from build123d import *

# Parameters (mm, degrees)
ESQUISSE3_R                  = 50
ESQUISSE3_R_2                = 42.5
BOSS_EXTRU_2_DEPTH           = 18
BOSS_EXTRU_3_START           = 3
ESQUISSE4_R                  = 50
BOSS_EXTRU_3_DEPTH           = 3
ESQUISSE5_R                  = 14
BOSS_EXTRU_4_DEPTH           = 7.5
BOSS_EXTRU_5_DEPTH           = 45
BOSS_EXTRU_5_DEPTH_BACK      = 45
CONG_1_R                     = 2
ESQUISSE6_R                  = 3.5
ENL_V_MAT_EXTRU_1_DEPTH      = 85.356386836
ESQUISSE7_R                  = 2
ENL_V_MAT_EXTRU_2_DEPTH      = 89.669329534
ENL_V_MAT_EXTRU_3_DEPTH      = 83.758685345
ENL_V_MAT_EXTRU_3_DEPTH_BACK = 4
ESQUISSE8_R                  = 3.5
ESQUISSE11_W                 = 24.696960071
ESQUISSE11_H                 = 3
BOSS_EXTRU_6_DEPTH           = 43
ENL_V_MAT_EXTRU_4_DEPTH      = 43
ESQUISSE13_R                 = 1.5
ENL_V_MAT_EXTRU_5_DEPTH      = 100.724620832
CHANFREIN1_SIZE              = 2
CHANFREIN2_SIZE              = 1.5


with BuildPart() as part:
    # Esquisse3 → Boss.-Extru.2 (new body)
    with BuildSketch(Plane(origin=(0, 0, 0), x_dir=(0, 0, -1), z_dir=(1, 0, 0))):
        Circle(ESQUISSE3_R)
        Circle(ESQUISSE3_R_2, mode=Mode.SUBTRACT)
    extrude(amount=BOSS_EXTRU_2_DEPTH)

    # Esquisse4 → Boss.-Extru.3 (add)
    with BuildSketch(Plane.ZY.offset(BOSS_EXTRU_3_START)):
        Circle(ESQUISSE4_R)
    extrude(amount=-BOSS_EXTRU_3_DEPTH)

    # Esquisse5 → Boss.-Extru.4 (add)
    with BuildSketch(Plane(origin=(0, 0, 0), x_dir=(0, 0, -1), z_dir=(1, 0, 0))):
        with Locations(Location((0, 0, 0), (0, 0, 180))):
            Circle(ESQUISSE5_R)
    extrude(amount=BOSS_EXTRU_4_DEPTH)

    # Esquisse10 → Boss.-Extru.5 (add, two sides: drawn at the far end of the back side and taken through both)
    with BuildSketch(Plane(origin=(0, 0, 0), x_dir=(1, 0, 0), z_dir=(0, 1, 0)).offset(-BOSS_EXTRU_5_DEPTH_BACK)):
        Polygon((-46, 23), (-3, 23), (-3, 20), (-43, 20), (-43, -20), (-3, -20), (-3, -23), (-46, -23), align=None)
    extrude(amount=BOSS_EXTRU_5_DEPTH + BOSS_EXTRU_5_DEPTH_BACK)

    # Congé1
    # the kernel refuses this fillet: 2 mm, written as the material it takes off along each edge
    with BuildSketch(Plane(origin=(-51, -45, -23), x_dir=(0, 0, 1), z_dir=(1, 0, 0)), Plane(origin=(-3, 45, 23), x_dir=(0, -1, 0), z_dir=(-1, 0, 0))) as cong_1_piece_1:
        with BuildLine():
            CenterArc((CONG_1_R, -CONG_1_R), CONG_1_R, 90, 90)
            Line((0, -CONG_1_R), (0, 0))
            Line((0, 0), (CONG_1_R, 0))
        make_face()
    extrude(amount=48, mode=Mode.SUBTRACT)
    with BuildSketch(Plane(origin=(-3, -45, 23), x_dir=(0, 1, 0), z_dir=(-1, 0, 0)), Plane(origin=(-51, 45, -23), x_dir=(0, 0, 1), z_dir=(1, 0, 0))) as cong_1_piece_2:
        with BuildLine():
            CenterArc((CONG_1_R, CONG_1_R), CONG_1_R, 180, 90)
            Line((0, CONG_1_R), (0, 0))
            Line((0, 0), (CONG_1_R, 0))
        make_face()
    extrude(amount=48, mode=Mode.SUBTRACT)

    # Esquisse6 → Enlèv. mat.-Extru.1 (cut, through all)
    with BuildSketch(Plane(origin=(0, 0, 0), x_dir=(0, 0, -1), z_dir=(1, 0, 0))):
        with Locations((-12.374368671, 12.374368671)):
            Circle(ESQUISSE6_R)
        with Locations((12.374368671, 12.374368671)):
            Circle(ESQUISSE6_R)
        with Locations((12.374368671, -12.374368671)):
            Circle(ESQUISSE6_R)
        with Locations((-12.374368671, -12.374368671)):
            Circle(ESQUISSE6_R)
    extrude(amount=-ENL_V_MAT_EXTRU_1_DEPTH, mode=Mode.SUBTRACT)

    # Esquisse7 → Enlèv. mat.-Extru.2 (cut, through all)
    with BuildSketch(Plane(origin=(7.5, 0, 0), x_dir=(0, 0, -1), z_dir=(1, 0, 0))):
        with Locations((0, 8.5)):
            Circle(ESQUISSE7_R)
        with Locations((7.361215932, 4.25)):
            Circle(ESQUISSE7_R)
        with Locations((7.361215932, -4.25)):
            Circle(ESQUISSE7_R)
        with Locations((0, -8.5)):
            Circle(ESQUISSE7_R)
        with Locations((-7.361215932, -4.25)):
            Circle(ESQUISSE7_R)
        with Locations((-7.361215932, 4.25)):
            Circle(ESQUISSE7_R)
    extrude(amount=-ENL_V_MAT_EXTRU_2_DEPTH, mode=Mode.SUBTRACT)

    # Esquisse8 → Enlèv. mat.-Extru.3 (cut, two sides: drawn at the far end of the back side and taken through both)
    with BuildSketch(Plane.ZY.offset(3).offset(-ENL_V_MAT_EXTRU_3_DEPTH_BACK)):
        with Locations((0, -8.5)):
            Circle(ESQUISSE8_R)
        with Locations((7.361215932, -4.25)):
            Circle(ESQUISSE8_R)
        with Locations((0, 8.5)):
            Circle(ESQUISSE8_R)
        with Locations((7.361215932, 4.25)):
            Circle(ESQUISSE8_R)
        with Locations((-7.361215932, -4.25)):
            Circle(ESQUISSE8_R)
        with Locations((-7.361215932, 4.25)):
            Circle(ESQUISSE8_R)
    extrude(amount=ENL_V_MAT_EXTRU_3_DEPTH + ENL_V_MAT_EXTRU_3_DEPTH_BACK, mode=Mode.SUBTRACT)

    # Esquisse11 → Boss.-Extru.6 (add)
    with BuildSketch(Plane.ZY.offset(3)):
        with Locations((35.348480036, 13.5)):
            Rectangle(ESQUISSE11_W, ESQUISSE11_H)
        with Locations((35.348480036, -13.5)):
            Rectangle(ESQUISSE11_W, ESQUISSE11_H)
        with Locations((-35.348480036, -13.5)):
            Rectangle(ESQUISSE11_W, ESQUISSE11_H)
        with Locations((-35.348480036, 13.5)):
            Rectangle(ESQUISSE11_W, ESQUISSE11_H)
    extrude(amount=BOSS_EXTRU_6_DEPTH)

    # Esquisse12 → Enlèv. mat.-Extru.4 (cut)
    with BuildSketch(Plane.XZ.offset(15)):
        Polygon((-46, -23), (-3, -47.696960071), (-46, -47.696960071), align=None)
        Polygon((-46, 23), (-3, 47.696960071), (-46, 47.696960071), align=None)
    extrude(amount=-ENL_V_MAT_EXTRU_4_DEPTH, mode=Mode.SUBTRACT)

    # Esquisse13 → Enlèv. mat.-Extru.5 (cut, through all)
    with BuildSketch(Plane(origin=(0, 0, -23), x_dir=(-1, 0, 0), z_dir=(0, 0, -1))):
        with Locations((23, 30)):
            Circle(ESQUISSE13_R)
        with Locations((23, -30)):
            Circle(ESQUISSE13_R)
        with Locations((23, 0)):
            Circle(ESQUISSE13_R)
    extrude(amount=-ENL_V_MAT_EXTRU_5_DEPTH, mode=Mode.SUBTRACT)

    # Chanfrein1
    chanfrein1_edges = [part.edges().sort_by_distance(p)[0] for p in [
        (18, 0, 50),
        (18, 0, 42.5),
    ]]
    chamfer(chanfrein1_edges, length=CHANFREIN1_SIZE)

    # Chanfrein2
    chanfrein2_edges = [part.edges().sort_by_distance(p)[0] for p in [
        (7.5, 0, -14),
    ]]
    chamfer(chanfrein2_edges, length=CHANFREIN2_SIZE)


solid = part.part
Work out the finished part from the listing and answer in its coordinate system (mm). A direction names the side the tool comes from. Round coordinates to 2 decimals unless told otherwise and drop trailing zeros. Loops run counter-clockwise (first coordinate to the right, second up) from the corner with the lowest first, then second, coordinate; pieces in that order, holes last. Notation, with made-up numbers: M -7,37 L 23,37 A34 cw 23,68 Z; hole C -11.5,-16 d5. An arc over 180 degrees is marked long. One line per question, with ' | ' between items. Start each with the question number.
(1) For a pull along X with two mould halves and no side action, classify faces 1 (the face through (4.296, -6.517, 0.26)), 2 (the face through (-21.89, 31.01, -21.52)), 3 (the face through (-24.801, -13.521, -35.176)) as released by +X, released by -X, zero draft, split by the parting line, or undercut.
(2) Find the intervals of material crossed by line 1 (Z direction, x = -22, y = -34); line 2 (Y direction, x = -12, z = -38); line 3 (X direction, y = -23, z = -40), in increasing order.
(3) Flat-ended cylindrical pins translate along their axes: pin 1 Ø12 at (x, y) = (3, 21) entering from +Z; pin 2 Ø12 at (x, y) = (-25.5, -0.5) entering from +Z; pin 3 Ø1.5 at (x, z) = (-10, 38) entering from -Y; pin 4 Ø7.5 at (x, z) = (-29, 37.5) entering from +Y. Find the tip coordinate at first contact, or state that the pin passes through.
(4) A tool of negligible diameter and unlimited length cuts with its end or side. For faces 4 (the face through (-19, 15, 32)), 5 (the face through (-25, 29, -23)), 6 (the face through (-25, 0, -23)), 7 (the face through (-44.479, -4.096, 3.865)), 8 (the face through (-44, 45, 0)), from which of +Z, -Z, +X, -X, +Y, -Y can it reach the whole face along a straight path? Write none if from no direction.
(5) A cutting plane is placed at A-A on x = -6.5. Write down the section's boundary in (y, z).
(6) A cutting plane is placed at B-B on x = -23. Give the number of separate pieces and of enclosed holes in the cut face, plus the area to 3 significant figures.
Geometry check:
1) face 1: zero draft | face 2: undercut | face 3: released by -X
2) line 1: z = -23 to -20, 20 to 23 | line 2: y = -15 to -12, 12 to 15 | line 3: x = -3 to 18
3) pin 1: stops at z = 47.7 | pin 2: stops at z = 23 | pin 3: stops at y = -15 | pin 4: passes through
4) face 4: +Z, -X, +Y | face 5: -Z, -X, +Y | face 6: -Z, -X | face 7: -X | face 8: +Z, -Z, -X, +Y
5) outline: M -45,-21 A2 ccw -43,-23 L -15,-23 L -15,-45.69 L -12,-45.69 L -12,-23 L 12,-23 L 12,-45.69 L 15,-45.69 L 15,-23 L 43,-23 A2 ccw 45,-21 L 45,-20 L -45,-20 Z; M -45,20 L 45,20 L 45,21 A2 ccw 43,23 L 15,23 L 15,45.69 L 12,45.69 L 12,23 L -12,23 L -12,45.69 L -15,45.69 L -15,23 L -43,23 A2 ccw -45,21 Z
6) separate pieces: 8 | enclosed holes: 0 | area: 641 mm²
